```python
from build123d import *

# Parameters (mm, degrees)
BOSS_EXTRU_1_DEPTH       = 2.5
ENL_V_MAT_EXTRU_14_DEPTH = 10
JOYSTICK_R               = 13.5
ENL_V_MAT_EXTRU_2_DEPTH  = 2.5
ESQUISSE2_W              = 14
ESQUISSE2_H              = 10
ENL_V_MAT_EXTRU_3_DEPTH  = 10
CONG_1_R                 = 2
CONG_2_R                 = 2
ESQUISSE3_W              = 14
ESQUISSE3_H              = 10
ENL_V_MAT_EXTRU_4_DEPTH  = 10
CONG_3_R                 = 2
CONG_4_R                 = 2
ENL_V_MAT_EXTRU_8_DEPTH  = 10
ESQUISSE5_R              = 3
ESQUISSE5_R_2            = 3.25
ENL_V_MAT_EXTRU_9_DEPTH  = 10
ESQUISSE6_R              = 4
ENL_V_MAT_EXTRU_15_DEPTH = 10


with BuildPart() as part:
    # Esquisse1 → Boss.-Extru.1 (new body)
    with BuildSketch(Plane.XY):
        with BuildLine():
            Line((-89.203921136, 33.34478673), (79.966078864, 33.34478673))
            ThreePointArc((79.966078864, 33.34478673), (83.50161277, 31.880320636), (84.966078864, 28.34478673))
            Line((84.966078864, 28.34478673), (84.966078864, -15.88521327))
            ThreePointArc((84.966078864, -15.88521327), (80.572680581, -26.491814988), (69.966078864, -30.88521327))
            Line((69.966078864, -30.88521327), (-79.203921136, -30.88521327))
            ThreePointArc((-79.203921136, -30.88521327), (-89.810522854, -26.491814988), (-94.203921136, -15.88521327))
            Line((-94.203921136, -15.88521327), (-94.203921136, 28.34478673))
            ThreePointArc((-94.203921136, 28.34478673), (-92.739455042, 31.880320636), (-89.203921136, 33.34478673))
        make_face()
    extrude(amount=BOSS_EXTRU_1_DEPTH)

    # 12x12 Button → Enlèv. mat.-Extru.14 (cut)
    with BuildSketch(Plane.XY.offset(2.5)):
        with BuildLine():
            ThreePointArc((47.62517912, 0.314609491), (46.965240695, -0.322324083), (46.382477581, -1.030554452))
            ThreePointArc((46.382477581, -1.030554452), (36.687266101, -5.758353734), (46.387422405, -10.475999265))
            ThreePointArc((46.387422405, -10.475999265), (47.121070973, -11.343088385), (47.970121608, -12.097539697))
            ThreePointArc((47.970121608, -12.097539697), (52.846080853, -22.107917903), (57.722033666, -12.097536564))
            ThreePointArc((57.722033666, -12.097536564), (58.521539603, -11.393399627), (59.220393145, -10.589271343))
            ThreePointArc((59.220393145, -10.589271343), (69.146073474, -5.755216476), (59.220398192, -0.921151245))
            ThreePointArc((59.220398192, -0.921151245), (58.674503702, -0.275289323), (58.063482277, 0.309339821))
            ThreePointArc((58.063482276, 0.309339821), (52.849240894, 10.038221143), (47.62517912, 0.314609492))
        make_face()
    extrude(amount=-ENL_V_MAT_EXTRU_14_DEPTH, mode=Mode.SUBTRACT)

    # Joystick → Enlèv. mat.-Extru.2 (cut)
    with BuildSketch(Plane.XY.offset(2.5)):
        with Locations((-68.703921136, -6.32521327)):
            Circle(JOYSTICK_R)
    extrude(amount=-ENL_V_MAT_EXTRU_2_DEPTH, mode=Mode.SUBTRACT)

    # Esquisse2 → Enlèv. mat.-Extru.3 (cut)
    with BuildSketch(Plane.XY.offset(2.5)):
        with Locations((53.056078864, 28.34478673)):
            Rectangle(ESQUISSE2_W, ESQUISSE2_H)
    extrude(amount=-ENL_V_MAT_EXTRU_3_DEPTH, mode=Mode.SUBTRACT)

    # Congé1
    cong_1_edges = [part.edges().sort_by_distance(p)[0] for p in [
        (46.056078864, 33.34478673, 1.25),
    ]]
    fillet(cong_1_edges, radius=CONG_1_R)

    # Congé2
    cong_2_edges = [part.edges().sort_by_distance(p)[0] for p in [
        (60.056078864, 33.34478673, 1.25),
    ]]
    fillet(cong_2_edges, radius=CONG_2_R)

    # Esquisse3 → Enlèv. mat.-Extru.4 (cut)
    with BuildSketch(Plane.XY.offset(2.5)):
        with Locations((-63.103921136, 28.34478673)):
            Rectangle(ESQUISSE3_W, ESQUISSE3_H)
    extrude(amount=-ENL_V_MAT_EXTRU_4_DEPTH, mode=Mode.SUBTRACT)

    # Congé3
    cong_3_edges = [part.edges().sort_by_distance(p)[0] for p in [
        (-70.103921136, 33.34478673, 1.25),
    ]]
    fillet(cong_3_edges, radius=CONG_3_R)

    # Congé4
    cong_4_edges = [part.edges().sort_by_distance(p)[0] for p in [
        (-56.103921136, 33.34478673, 1.25),
    ]]
    fillet(cong_4_edges, radius=CONG_4_R)

    # Esquisse4 → Enlèv. mat.-Extru.8 (cut)
    with BuildSketch(Plane.XY.offset(2.5)):
        with BuildLine():
            Line((63.848163441, 19.991775112), (79.478036154, 24.706585194))
            ThreePointArc((79.478036154, 24.706585194), (80.785408643, 24.005170837), (80.083994286, 22.697798347))
            Line((80.083994286, 22.697798347), (64.454121573, 17.982988266))
            ThreePointArc((64.454121573, 17.982988266), (63.146749084, 18.684402623), (63.848163441, 19.991775112))
        make_face()
        with BuildLine():
            Line((63.539756046, 23.02230266), (78.059151304, 27.402133027))
            ThreePointArc((78.059151304, 27.402133027), (79.327394653, 26.721711723), (78.646973349, 25.453468374))
            Line((78.646973349, 25.453468374), (64.127578092, 21.073638007))
            ThreePointArc((64.127578092, 21.073638007), (62.859334743, 21.754059311), (63.539756046, 23.02230266))
        make_face()
        with BuildLine():
            Line((64.721267087, 26.554024385), (75.121728293, 29.691362753))
            ThreePointArc((75.121728293, 29.691362753), (76.350895216, 29.031906221), (75.691438685, 27.802739299))
            Line((75.691438685, 27.802739299), (65.290977478, 24.665400931))
            ThreePointArc((65.290977478, 24.665400931), (64.061810556, 25.324857462), (64.721267087, 26.554024385))
        make_face()
        with BuildLine():
            Line((65.314724126, 17.237366416), (79.779269942, 21.600651242))
            ThreePointArc((79.779269942, 21.600651242), (81.126757031, 20.877715126), (80.403820915, 19.530228036))
            Line((80.403820915, 19.530228036), (65.939275099, 15.166943211))
            ThreePointArc((65.939275099, 15.166943211), (64.591788009, 15.889879327), (65.314724126, 17.237366416))
        make_face()
        with BuildLine():
            Line((68.322797362, 14.963301678), (78.530507851, 18.042496065))
            ThreePointArc((78.530507851, 18.042496065), (79.931361718, 17.290928304), (79.179793957, 15.890074436))
            Line((79.179793957, 15.890074436), (68.972083468, 12.810880049))
            ThreePointArc((68.972083468, 12.810880049), (67.571229601, 13.562447811), (68.322797362, 14.963301678))
        make_face()
    extrude(amount=-ENL_V_MAT_EXTRU_8_DEPTH, mode=Mode.SUBTRACT)

    # Esquisse5 → Enlèv. mat.-Extru.9 (cut)
    with BuildSketch(Plane.XY.offset(2.5)):
        with Locations((76.346078864, -22.88521327)):
            Circle(ESQUISSE5_R)
        with Locations((-86.203921136, -23.53521327)):
            Circle(ESQUISSE5_R)
        with Locations((76.346078864, 5.34478673)):
            Circle(ESQUISSE5_R)
        with Locations((-60.233921136, 13.83478673)):
            Circle(ESQUISSE5_R)
        with Locations((-87.483921136, -15.91521327)):
            Circle(ESQUISSE5_R_2)
        with Locations((39.756078864, 26.62478673)):
            Circle(ESQUISSE5_R_2)
        with Locations((46.496078864, 17.10478673)):
            Circle(ESQUISSE5_R_2)
    extrude(amount=-ENL_V_MAT_EXTRU_9_DEPTH, mode=Mode.SUBTRACT)

    # Esquisse6 → Enlèv. mat.-Extru.15 (cut)
    with BuildSketch(Plane.XY.offset(2.5)):
        with Locations((-96.703921136, -4.38521327)):
            Circle(ESQUISSE6_R)
        with Locations((-96.703921136, 23.15478673)):
            Circle(ESQUISSE6_R)
        with Locations((87.466078864, -6.16521327)):
            Circle(ESQUISSE6_R)
    extrude(amount=-ENL_V_MAT_EXTRU_15_DEPTH, mode=Mode.SUBTRACT)


solid = part.part
```
Here's how the part is built. I have some questions about the finished solid (model axes, mm). A direction names the side the tool comes from. Coordinates: 2 decimals unless noted, no trailing zeros. Write each loop counter-clockwise with the first axis right and the second up, starting at its lowest first coordinate (ties: lowest second). Pieces come first, ordered by that corner, then holes. Notation, with made-up numbers: (-11, 73) -> (2, 73) arc R29 cw to (2, 107) -> close; hole circle Ø7 at (86.25, -15). An arc over 180 degrees is marked (long way). Use a Markdown table: item, result. Add a question column.
(1) I'm going to push a flat-ended pin straight in: P1, Ø0.8, axis at y = 25.5, z = 1.5, coming from the -X side. Where does the tip first touch, or does it pass through?
(2) We'd pull the mould along X, two halves only. Please class faces 3 (the flat face through (-3, 2, 2.5)), 4 (the cylindrical face through (83.46, 31.92, 1.23)), 5 (the cylindrical face through (36.69, -5.57, 1.27)), 6 (the cylindrical face through (-89.7, -26.6, 1.2)): +X half, -X half, draft (parallel to the pull), parting line (faces both ways), or undercut.
(3) If we section it at B-B, the plane z = 1.3: State how many separate pieces and enclosed holes the cut face has, and give its area (3 significant figures).
(4) For faces 1 (the cylindrical face through (80.689, -26.375, 1.232)), 2 (the flat face through (70.564, 26.256, 1.268)), which set-ups out of +Z, -Z, +X, -X, +Y, -Y let a thin tool reach every point of the face, with its end or its side?
(5) If we section it at A-A, the plane x = 40: Write out the boundary of the cut face in (y, z), and give its area (3 significant figures).
(6) Please list where these lines run through material, in increasing order: line 1 (X direction, y = -18, z = 0.95); line 2 (Y direction, x = 66.5, z = 2.15); line 3 (X direction, y = -3, z = 2.35).
Outcome:
| question | item | result |
|---|---|---|
| 1 | P1 | stops at x = -93.79 |
| 2 | face 3 | draft |
| 2 | face 4 | +X half |
| 2 | face 5 | undercut |
| 2 | face 6 | -X half |
| 3 | separate pieces | 1 |
| 3 | enclosed holes | 14 |
| 3 | area | 9,590 mm^2 |
| 4 | face 1 | +Z, -Z, +X, -Y |
| 4 | face 2 | +Z, -Z |
| 5 | outline | (-30.89, 0) -> (-11.12, 0) -> (-11.12, 2.5) -> (-30.89, 2.5) -> close; (-0.39, 0) -> (23.38, 0) -> (23.38, 2.5) -> (-0.39, 2.5) -> close; (29.87, 0) -> (33.34, 0) -> (33.34, 2.5) -> (29.87, 2.5) -> close |
| 5 | area | 118 mm^2 |
| 6 | line 1 | x = -94.05 to -89.98, -84.99 to -75.48, -61.93 to 47.01, 58.68 to 84.82 |
| 6 | line 2 | y = -30.89 to -10.8, -0.71 to 15.34, 17.59 to 18.6, 20.79 to 21.79, 23.92 to 25.03, 27.09 to 33.34 |
| 6 | line 3 | x = -92.95 to -81.79, -55.62 to 37.36, 68.49 to 84.97 |
